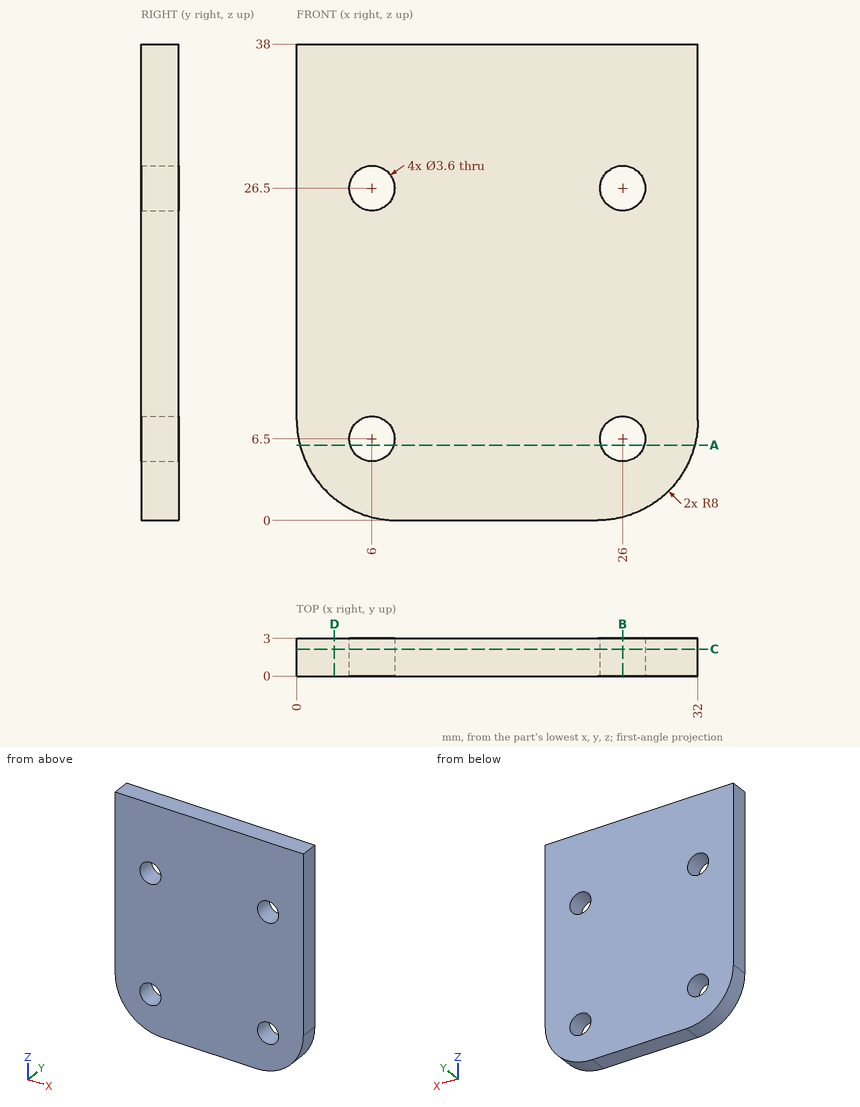
The drawing under review shows one solid part. Ordinate dimensions are in mm from its lowest x, y, z. Round coordinates to 2 decimals unless told otherwise and drop trailing zeros. Order: outer loops, then holes, each group sorted by start corner. A loop starts at its lowest first (then second) coordinate and runs counter-clockwise, first axis right, second up. Notation, with made-up numbers: (29, 0) -> (40, 0) arc R31 cw to (40, 26) -> close; hole circle Ø10 at (75, 11.5). An arc over 180 degrees is marked (long way). Use a Markdown table: item, result.
Item 1: Take a section at C-C (y = 2.15). State the section outline as (x, z) points.
Resolved:
| item | result |
|---|---|
| outline | (0, 8) arc R8 ccw to (8, 0) -> (24, 0) arc R8 ccw to (32, 8) -> (32, 38) -> (0, 38) -> close; hole circle Ø3.6 at (6, 6.5); hole circle Ø3.6 at (6, 26.5); hole circle Ø3.6 at (26, 6.5); hole circle Ø3.6 at (26, 26.5) |
Item 2: Take a section at A-A (z = 6). State the section outline as (x, y) points, plus the area to 3 significant figures.
Resolved:
| item | result |
|---|---|
| outline | (0.25, 0) -> (4.27, 0) -> (4.27, 3) -> (0.25, 3) -> close; (7.73, 0) -> (24.27, 0) -> (24.27, 3) -> (7.73, 3) -> close; (27.73, 0) -> (31.75, 0) -> (31.75, 3) -> (27.73, 3) -> close |
| area | 73.7 mm² |
Item 3: For line 1 along X through (y, z) = (0.7, 26.5); line 2 along Z through (x, y) = (6, 0.95); line 3 along Z through (x, y) = (27, 2.2), list the stretches that pass through material, from the lowest coordinate up. Write a range as [from, to].
Resolved:
| item | result |
|---|---|
| line 1 | x = [0, 4.2], [7.8, 24.2], [27.8, 32] |
| line 2 | z = [0.25, 4.7], [8.3, 24.7], [28.3, 38] |
| line 3 | z = [0.58, 5], [8, 25], [28, 38] |
Item 4: Take a section at B-B (x = 26). State the section outline as (y, z) points.
Resolved:
| item | result |
|---|---|
| outline | (0, 0.25) -> (3, 0.25) -> (3, 4.7) -> (0, 4.7) -> close; (0, 8.3) -> (3, 8.3) -> (3, 24.7) -> (0, 24.7) -> close; (0, 28.3) -> (3, 28.3) -> (3, 38) -> (0, 38) -> close |
Item 5: Take a section at D-D (x = 3). State the section outline as (y, z) points (3 decimals).
Resolved:
| item | result |
|---|---|
| outline | (0, 1.755) -> (3, 1.755) -> (3, 38) -> (0, 38) -> close |
